Job drawing, mm, ordinate dimensions from the low corner. One solid piece. A direction names the side the tool comes from. Round coordinates to 2 decimals unless told otherwise and drop trailing zeros. Loops run counter-clockwise (first coordinate to the right, second up) from the corner with the lowest first, then second, coordinate; pieces in that order, holes last. Notation, with made-up numbers: (29.25, 72.25) - (78.25, 72.25) arc R14 ccw to (78.25, 85.25) - close; hole circle Ø5 at (22, -3.75). An arc over 180 degrees is marked (long way). Answer as CSV lines item,"result". Start each with the question number.
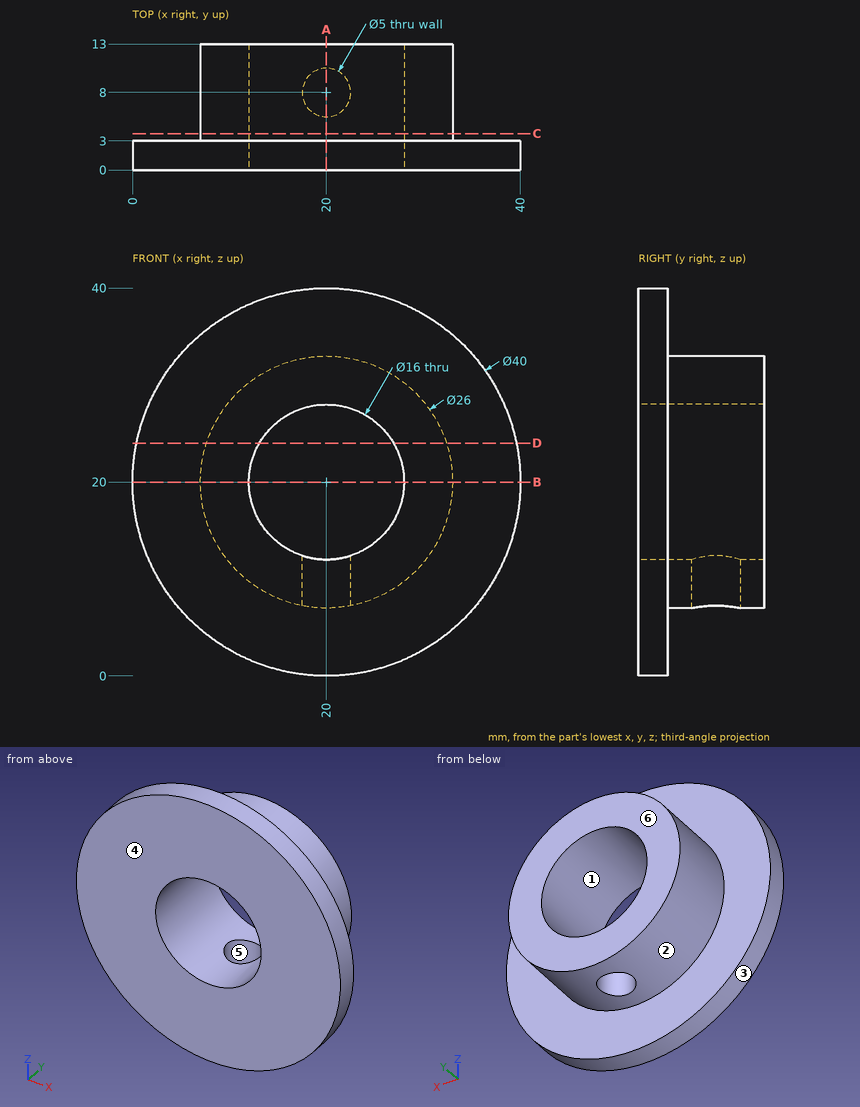
Q1. Band-saw the part on A-A, the plane x = 20. List the corners of the cut face in (y, z), then the cut area to 3 significant figures.
Q2. Band-saw the part on D-D, the plane z = 24. List the corners of the cut face in (x, y).
Q3. Pin check, flat tips, straight feed: pin 1 Ø13 at (x, z) = (20, 20) entering from -Y; pin 2 Ø6 at (x, y) = (9.5, 1.5) entering from +Z; pin 3 Ø5 at (y, z) = (7.5, 28) entering from -X; pin 4 Ø5 at (y, z) = (8.5, 22.5) entering from -X. Stop position of each tip, or through.
Q4. Tool access for the marked faces 1 and 2: list every direction of +Z, -Z, +X, -X, +Y, -Y with a clear straight run to the whole face (end or side of a thin tool).
Q5. Band-saw the part on B-B, the plane z = 20. List the corners of the cut face in (x, y), then the cut area to 3 significant figures.
Q6. Wall check: probe 1 along X at (y, z) = (8, 20); probe 2 along Y at (x, z) = (5, 18); probe 3 along X at (y, z) = (7, 10). Give the ranges that are in metal, low to high. Write a range as [from, to].
Q7. Band-saw the part on C-C, the plane y = 3.75. List the corners of the cut face in (x, z).
Q8. Two-plate mould, pull along Y, no slides. Class the marked faces 3, 4, 5 and 6: released by +Y, released by -Y, zero draft, split by the parting line, or undercut.
Reported:
1,outline,"(0, 0) - (3, 0) - (3, 7) - (5.5, 7) - (5.5, 12) - (0, 12) - close; (0, 28) - (13, 28) - (13, 33) - (3, 33) - (3, 40) - (0, 40) - close; (10.5, 7) - (13, 7) - (13, 12) - (10.5, 12) - close"
1,area,"147 mm2"
2,outline,"(0.4, 0) - (13.07, 0) - (13.07, 13) - (7.63, 13) - (7.63, 3) - (0.4, 3) - close; (26.93, 0) - (39.6, 0) - (39.6, 3) - (32.37, 3) - (32.37, 13) - (26.93, 13) - close"
3,pin 1,"passes through"
3,pin 2,"stops at z = 38.54"
3,pin 3,"stops at x = 8.22"
3,pin 4,"stops at x = 7"
4,face 1,"+Y, -Y"
4,face 2,"+Y"
5,outline,"(0, 0) - (12, 0) - (12, 13) - (7, 13) - (7, 3) - (0, 3) - close; (28, 0) - (40, 0) - (40, 3) - (33, 3) - (33, 13) - (28, 13) - close"
5,area,"172 mm2"
6,probe 1,"x = [7, 12], [28, 33]"
6,probe 2,"y = [0, 3]"
6,probe 3,"x = [11.69, 17.71], [22.29, 28.31]"
7,outline,"circle Ø26 at (20, 20); hole circle Ø16 at (20, 20)"
8,face 3,"zero draft"
8,face 4,"released by -Y"
8,face 5,"undercut"
8,face 6,"released by +Y"
